```python
from build123d import *

# Parameters (mm, degrees)
POCKET_DEPTH         = 0.001
POCKET_DEPTH_BACK    = 6.001
POCKET001_DEPTH      = 0.001
POCKET001_DEPTH_BACK = 6.001


with BuildPart() as part:
    # AdditivePipe: sweep along a path in Sketch
    with BuildLine(Plane.XY) as additivepipe_path:
        ThreePointArc((240, 0), (221.731088, 91.844024), (169.705627, 169.705627))
    # Sketch001 → AdditivePipe (sweep)
    with BuildSketch(Plane(origin=(240, 0, 0), x_dir=(1, 0, 0), z_dir=(0, -1, 0))):
        Polygon((-8, 0), (8, 0), (8, 1), (1, 1), (1, 6), (-1, 6), (-1, 1), (-8, 1), align=None)
    sweep(path=additivepipe_path.line, is_frenet=True)

    # Sketch002 → Pocket (cut, two sides)
    with BuildSketch(Plane.XY) as pocket_sk:
        Polygon((235.663538, 6.38431), (236.75, 0), (243.25, 0), (244.16042, 6.614498), align=None)
    extrude(amount=-POCKET_DEPTH, mode=Mode.SUBTRACT)
    extrude(pocket_sk.sketch, amount=POCKET_DEPTH_BACK, mode=Mode.SUBTRACT)

    # Sketch003 → Pocket001 (cut, two sides)
    with BuildSketch(Plane.XY) as pocket001_sk:
        Polygon((166.8772, 166.8772), (171.721217, 163.342657), (155.73217, 148.133741), (152.027958, 152.027958), align=None)
        Polygon((172.534055, 172.534055), (176.06859, 167.477914), (192.057638, 182.68683), (187.383297, 187.383297), align=None)
    extrude(amount=-POCKET001_DEPTH, mode=Mode.SUBTRACT)
    extrude(pocket001_sk.sketch, amount=POCKET001_DEPTH_BACK, mode=Mode.SUBTRACT)


solid = part.part
```
Design review of the part built by this model. Coordinates are the model's own, in mm. A direction names the side the tool comes from. Give positions to 0.01 mm unless a question says otherwise; leave off trailing zeros. Order: outer loops, then holes, each group sorted by start corner. A loop starts at its lowest first (then second) coordinate and runs counter-clockwise, first axis right, second up. Notation, with made-up numbers: (-9.5, 82) -> (45.5, 82) arc R24 cw to (45.5, 105) -> close; hole circle Ø7 at (36, -10). An arc over 180 degrees is marked (long way). Write item = value, one per line. Start each with the question number.
(1) Mouldability with a two-part tool opening along X and no side actions: class faces 5 (the face through (221.888, 94.057, 3.535)), 6 (the face through (174.277, 170.041, 0.493)), 7 (the face through (170, 170, 2)) as +X half, -X half, draft (parallel to the pull), parting line (faces both ways), or undercut.
(2) For pin 1 (1 mm diameter, centred on y = 155, z = 3, fed in from -X), flat-tipped, find the tip position at first contact; note if it passes through.
(3) We need section C-C on z = 4.95. Write out the cut boundary in (x, y), plus the area to 3 significant figures.
(4) To check wall thickness, follow line 1 along Z through (x, y) = (229, 53); line 2 along X through (y, z) = (105.5, 1.3); line 3 along Y through (x, z) = (210, 4.45). State the ranges of each line that lie inside material, in increasing order.
(5) We need section A-A on y = 82.5. Write out the cut boundary in (x, z), plus the area to 3 significant figures.
(6) For faces 1 (the face through (177.855, 169.177, 0.493)), 2 (the face through (226, 92, 1)), 3 (the face through (216, 90, 1)), 4 (the face through (169.935, 161.644, 0.493)), list the 3-axis set-ups (+Z, -Z, +X, -X, +Y, -Y) from which the entire face can be reached by the end or side of a thin tool; tool diameter is ignored.
(7) We need section B-B on x = 207.5. Write out the cut boundary in (y, z).
Numbers:
q1.face_5 = +X half
q1.face_6 = undercut
q1.face_7 = -X half
q2.pin_1 = 181.5
q3.outline = (169, 169) arc R239 cw to (238.91, 6.47) -> (240.91, 6.53) arc R241 ccw to (170.41, 170.41) -> close
q3.area = 364 mm^2
q4.line_1 = 0 to 1
q4.line_2 = 214.45 to 216.68
q4.line_3 = 114.11 to 118.24
q5.outline = (216.84, 0) -> (233.88, 0) -> (233.88, 1) -> (226.44, 1) -> (226.44, 6) -> (224.31, 6) -> (224.31, 1) -> (216.84, 1) -> close
q5.area = 27.7 mm^2
q6.face_1 = +Z, -Z, +Y
q6.face_2 = +Z, +X, +Y
q6.face_3 = +Z, -X, -Y
q6.face_4 = +Z, -Z, -X
q7.outline = (103.77, 0) -> (135.82, 0) -> (135.82, 1) -> (122.58, 1) -> (122.58, 6) -> (118.59, 6) -> (118.59, 1) -> (103.77, 1) -> close
